from build123d import *

# Parameters (mm, degrees)
BOSS_EXTRUDE1_DEPTH = 3


with BuildPart() as part:
    # Sketch1 → Boss-Extrude1 (new body)
    with BuildSketch(Plane.XY):
        with BuildLine():
            Line((-4.955370371, 4.8), (-7.955370371, 4.8))
            Line((-7.955370371, 4.8), (-7.955370371, 9.6))
            Line((-7.955370371, 9.6), (-4.955370371, 9.6))
            Line((-4.955370371, 9.6), (-4.955370371, 14.4))
            Line((-4.955370371, 14.4), (-7.955370371, 14.4))
            Line((-7.955370371, 14.4), (-7.955370371, 19.2))
            Line((-7.955370371, 19.2), (-4.955370371, 19.2))
            Line((-4.955370371, 19.2), (-4.955370371, 24))
            Line((-4.955370371, 24), (30.844629629, 24))
            Line((30.844629629, 24), (30.844629629, 27))
            Line((30.844629629, 27), (66.644629629, 27))
            Line((66.644629629, 27), (66.644629629, 24))
            Line((66.644629629, 24), (102.444629629, 24))
            Line((102.444629629, 24), (102.444629629, 27))
            Line((102.444629629, 27), (138.244629629, 27))
            Line((138.244629629, 27), (138.244629629, 24))
            Line((138.244629629, 24), (174.044629629, 24))
            Line((174.044629629, 24), (174.044629629, 19.2))
            Line((174.044629629, 19.2), (177.044629629, 19.2))
            Line((177.044629629, 19.2), (177.044629629, 14.4))
            Line((177.044629629, 14.4), (174.044629629, 14.4))
            Line((174.044629629, 14.4), (174.044629629, 9.6))
            Line((174.044629629, 9.6), (177.044629629, 9.6))
            Line((177.044629629, 9.6), (177.044629629, 4.8))
            Line((177.044629629, 4.8), (174.044629629, 4.8))
            Line((174.044629629, 4.8), (174.044629629, 0))
            Line((174.044629629, 0), (138.244629629, 0))
            Line((138.244629629, 0), (138.244629629, -3))
            Line((138.244629629, -3), (112.794629629, -3))
            Line((112.794629629, -3), (112.794629629, 0))
            Line((112.794629629, 0), (112.794629629, 6))
            ThreePointArc((112.794629629, 6), (107.794629629, 11), (102.794629629, 6))
            Line((102.794629629, 6), (102.794629629, 0))
            Line((102.794629629, 0), (102.444629629, 0))
            Line((102.444629629, 0), (66.644629629, 0))
            Line((66.644629629, 0), (66.644629629, -3))
            Line((66.644629629, -3), (32.794629629, -3))
            Line((32.794629629, -3), (32.794629629, 6))
            ThreePointArc((32.794629629, 6), (27.794629629, 11), (22.794629629, 6))
            Line((22.794629629, 6), (22.794629629, 0))
            Line((22.794629629, 0), (-4.955370371, 0))
            Line((-4.955370371, 0), (-4.955370371, 4.8))
        make_face()
    extrude(amount=BOSS_EXTRUDE1_DEPTH)


solid = part.part
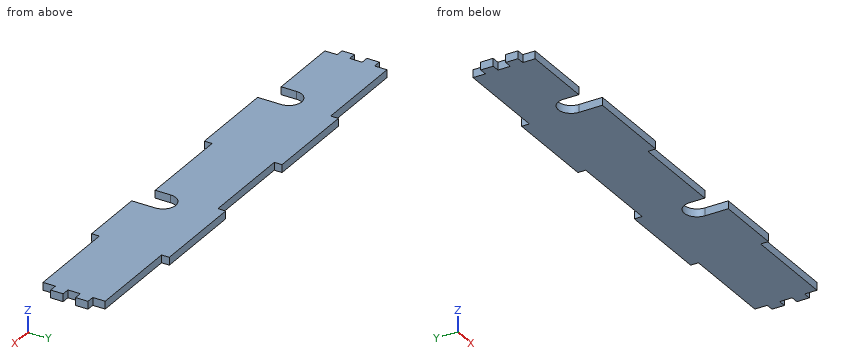
Input: part model. Units: mm. Frame: model coordinates. Coordinates: 2 decimals unless noted, no trailing zeros. Write each loop counter-clockwise with the first axis right and the second up, starting at its lowest first coordinate (ties: lowest second). Pieces come first, ordered by that corner, then holes. Notation, with made-up numbers: M 74,-34.75 L 91,-34.75 A29 ccw 91,-1.75 Z; hole C -20,-35 d9. An arc over 180 degrees is marked long. Answer as a JSON object with one key per item and string values. Group by question number.
(1) Section A-A on y = 2.5. Output: boundary loops of the cut face in (x, z).
(2) Section B-B on x = 80.5. Output: boundary loops of the cut face in (y, z), plus the area to 3 significant figures.
(3) Contact query for flat-ended pins moving along their axis: P1, Ø0.9, axis at y = -1, z = 1.5, coming from the +X side; P2, Ø1.5, axis at x = 9.5, z = 1.5, coming from the -Y side; P3, Ø1.5, axis at x = 90.5, z = 1, coming from the +Y side. Output: stop coordinate, or through.
(4) Ray query, line 1 along X through (y, z) = (0.25, 0.55); line 2 along X through (y, z) = (6.25, 0.75); line 3 along X through (y, z) = (25, 1.4). Return the intervals inside material, ascending. Write a range as [from, to].
Result set:
{
 "1": {"outline": "M -4.96,0 L 22.79,0 L 22.79,3 L -4.96,3 Z; M 32.79,0 L 102.79,0 L 102.79,3 L 32.79,3 Z; M 112.79,0 L 174.04,0 L 174.04,3 L 112.79,3 Z"},
 "2": {"outline": "M 0,0 L 24,0 L 24,3 L 0,3 Z", "area": "72.0 mm2"},
 "3": {"P1": "stops at x = 138.24", "P2": "stops at y = 0", "P3": "stops at y = 24"},
 "4": {"line 1": "x = [-4.96, 22.79], [32.79, 102.79], [112.79, 174.04]", "line 2": "x = [-7.96, 22.8], [32.79, 102.8], [112.79, 177.04]", "line 3": "x = [30.84, 66.64], [102.44, 138.24]"}
}
